Model file for the job. Use its own axes, mm. A direction names the side the tool comes from. Give positions to 0.01 mm unless a question says otherwise; leave off trailing zeros. Order: outer loops, then holes, each group sorted by start corner. A loop starts at its lowest first (then second) coordinate and runs counter-clockwise, first axis right, second up. Notation, with made-up numbers: (42, -17) -> (88, -17) arc R32 ccw to (88, 21) -> close; hole circle Ø6 at (-15, 32.5). An arc over 180 degrees is marked (long way). Use CSV: the item, a comma, the result in double quotes. Start each with the question number.
1. Cut at B-B on x = 33.5. List the corners of the cut face in (y, z).
2. Wall check: line 1 (Z direction, x = 36, y = -17); line 2 (X direction, y = -14, z = 18); line 3 (X direction, y = -5.5, z = 34). Give the ranges that are in metal, low to high. Write a range as from..to.
3. Cut at D-D on x = 4. List the corners of the cut face in (y, z), then the cut area to 3 significant figures.
4. Pull direction Y, two halves, no side cores. Call faces 3 (the flat face through (50.8, -13, 19)), 4 (the cylindrical face through (25.684, -1.528, 36.651)), 5 (the cylindrical face through (1.63, -12.807, 36.395)): released by +Y, released by -Y, zero draft, split by the parting line, or undercut.
5. Cut at A-A on y = -14.5. List the corners of the cut face in (x, z).
6. Cut at C-C on z = 24.5. List the corners of the cut face in (x, y), then the cut area to 3 significant figures.
7. Drop flat-ended pins along their axis: pin 1 (14 mm diameter, centred on x = 21.5, z = 16, fed in from -Y); pin 2 (6 mm diameter, centred on x = 5.5, z = 33.5, fed in from -Y); pin 3 (3 mm diameter, centred on y = -3, z = 29.5, fed in from -X). Give the stop position or say it passes through.
8. 3-axis set-ups, long thin cutter, end or side, ignore diameter. For faces 1 (the flat face through (25, -13, 38.1)), 2 (the cylindrical face through (25.684, -23.695, 1.63)): which of +Z, -Z, +X, -X, +Y, -Y reach the whole face in a straight line?
```python
from build123d import *

# Parameters (mm, degrees)
F0_W     = 50.8
F0_H     = 38.1
F1_DEPTH = 25.4
F2_R     = 5.08
F3_T     = -0.254


# Not quite as in the source:
# - a shell that OpenCascade refuses in one call is made with other operations: the cavity is built on its own and cut out


with BuildPart() as f1:
    # F0 (on Front) → F1 (new body)
    with BuildSketch(Plane.XZ):
        with Locations((25.4, 19.05)):
            Rectangle(F0_W, F0_H)
    extrude(amount=F1_DEPTH)

    # F2
    f2_edges = [f1.edges().sort_by_distance(p)[0] for p in [
        (50.8, -12.7, 38.1),
        (25.4, -25.4, 38.1),
        (25.4, 0, 38.1),
        (50.8, -25.4, 19.05),
        (50.8, 0, 19.05),
        (50.8, -12.7, 0),
        (25.4, -25.4, 0),
        (25.4, 0, 0),
        (0, -25.4, 19.05),
        (0, -12.7, 38.1),
        (0, -12.7, 0),
        (0, 0, 19.05),
    ]]
    fillet(f2_edges, radius=F2_R)

    # F3: a shell. OpenCascade refuses it in one call, so the cavity is built on its own and cut out:
    # the body offset inwards by the wall thickness, plus a prism from it out through each open face.
    f3_core = offset(f1.part, amount=F3_T, mode=Mode.PRIVATE)
    f3_exits = [f3_core.faces().sort_by_distance(p)[0] for p in [
        (25.4, -25.146, 19.05),
    ]]
    add(f3_core, mode=Mode.SUBTRACT)
    extrude(f3_exits, amount=-F3_T, mode=Mode.SUBTRACT)


solid = f1.part
```
Verdict:
1,outline,"(-25.4, 5.08) arc R5.08 ccw to (-20.32, 0) -> (-5.08, 0) arc R5.08 ccw to (0, 5.08) -> (0, 33.02) arc R5.08 ccw to (-5.08, 38.1) -> (-20.32, 38.1) arc R5.08 ccw to (-25.4, 33.02) -> (-25.15, 33.02) arc R4.83 cw to (-20.32, 37.85) -> (-5.08, 37.85) arc R4.83 cw to (-0.25, 33.02) -> (-0.25, 5.08) arc R4.83 cw to (-5.08, 0.25) -> (-20.32, 0.25) arc R4.83 cw to (-25.15, 5.08) -> close"
2,line 1,"0..0.25, 37.85..38.1"
2,line 2,"0..0.25, 50.55..50.8"
2,line 3,"0.1..0.35, 50.45..50.7"
3,outline,"(-25.28, 5.08) arc R4.96 ccw to (-20.32, 0.12) -> (-5.08, 0.12) arc R4.96 ccw to (-0.12, 5.08) -> (-0.12, 33.02) arc R4.96 ccw to (-5.08, 37.98) -> (-20.32, 37.98) arc R4.96 ccw to (-25.28, 33.02) -> close; hole (-25.02, 5.08) arc R4.7 ccw to (-20.32, 0.38) -> (-5.08, 0.38) arc R4.7 ccw to (-0.38, 5.08) -> (-0.38, 33.02) arc R4.7 ccw to (-5.08, 37.72) -> (-20.32, 37.72) arc R4.7 ccw to (-25.02, 33.02) -> close"
3,area,"30.4 mm^2"
4,face 3,"zero draft"
4,face 4,"released by +Y"
4,face 5,"undercut"
5,outline,"(0, 5.08) arc R5.08 ccw to (5.08, 0) -> (45.72, 0) arc R5.08 ccw to (50.8, 5.08) -> (50.8, 33.02) arc R5.08 ccw to (45.72, 38.1) -> (5.08, 38.1) arc R5.08 ccw to (0, 33.02) -> close; hole (0.25, 5.08) arc R4.83 ccw to (5.08, 0.25) -> (45.72, 0.25) arc R4.83 ccw to (50.55, 5.08) -> (50.55, 33.02) arc R4.83 ccw to (45.72, 37.85) -> (5.08, 37.85) arc R4.83 ccw to (0.25, 33.02) -> close"
6,outline,"(0, -20.32) arc R5.08 ccw to (5.08, -25.4) -> (5.08, -25.15) arc R4.83 cw to (0.25, -20.32) -> (0.25, -5.08) arc R4.83 cw to (5.08, -0.25) -> (45.72, -0.25) arc R4.83 cw to (50.55, -5.08) -> (50.55, -20.32) arc R4.83 cw to (45.72, -25.15) -> (45.72, -25.4) arc R5.08 ccw to (50.8, -20.32) -> (50.8, -5.08) arc R5.08 ccw to (45.72, 0) -> (5.08, 0) arc R5.08 ccw to (0, -5.08) -> close"
6,area,"26.0 mm^2"
7,pin 1,"y = -0.25"
7,pin 2,"y = -25.4"
7,pin 3,"x = 0.03"
8,face 1,"+Z, +X, -X, +Y, -Y"
8,face 2,"none"
